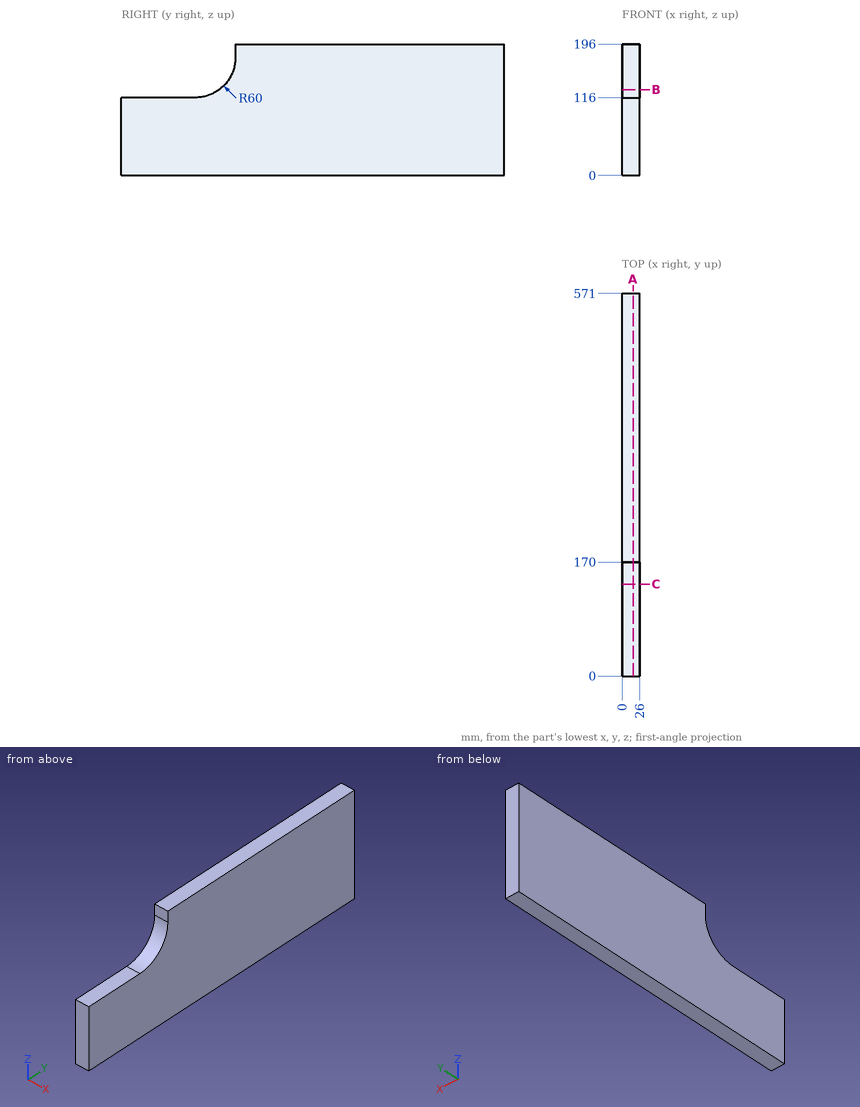
Job drawing, mm, ordinate dimensions from the low corner. One solid piece. Give positions to 0.01 mm unless a question says otherwise; leave off trailing zeros. Loops run counter-clockwise (first coordinate to the right, second up) from the corner with the lowest first, then second, coordinate; pieces in that order, holes last. Notation, with made-up numbers: M -37.5,83.25 L -10.5,83.25 A10 cw -10.5,101.25 Z; hole C -35.5,-3 d3. An arc over 180 degrees is marked long. Use one line per item in the form item = value.
Item 1: Drill centre lines: L1, parallel to Z at x = 8.5, y = 43; L2, parallel to Y at x = 24, z = 185; L3, parallel to Y at x = 4.25, z = 161. Where is each one in solid material? Low to high.
Filled in:
L1 = 0 to 116
L2 = 170 to 571
L3 = 168.09 to 571
Item 2: Slice it at B-B on z = 128. List the corners of the cut face in (x, y).
Filled in:
outline = M 0,146 L 26,146 L 26,571 L 0,571 Z
Item 3: Slice it at A-A on x = 16.5. List the corners of the cut face in (y, z), and give its area (3 significant figures).
Filled in:
outline = M 0,0 L 571,0 L 571,196 L 170,196 L 170,176 A60 cw 110,116 L 0,116 Z
area = 99,100 mm^2
Item 4: Flat gauge pins, fed straight in: pin 1 Ø10 at (x, z) = (9.5, 182.5) entering from -Y; pin 2 Ø8 at (x, y) = (16.5, 72) entering from +Z; pin 3 Ø5 at (x, z) = (13, 141) entering from -Y. Where does each tip first touch, or does it go through?
Filled in:
pin_1 = 170
pin_2 = 116
pin_3 = 156.84
Item 5: Slice it at C-C on y = 137. List the corners of the cut face in (x, z).
Filled in:
outline = M 0,0 L 26,0 L 26,122.42 L 0,122.42 Z
